Model file for the job. Use its own axes, mm. A direction names the side the tool comes from. Give positions to 0.01 mm unless a question says otherwise; leave off trailing zeros. Write each loop counter-clockwise with the first axis right and the second up, starting at its lowest first coordinate (ties: lowest second). Pieces come first, ordered by that corner, then holes. Notation, with made-up numbers: (59, 16) - (77, 16) arc R10 ccw to (77, 34) - close; hole circle Ø8 at (4.5, -14.5). An arc over 180 degrees is marked (long way). One line per item, written item: value. Start each with the question number.
(1) Drop flat-ended pins along their axis: P1, Ø4, axis at x = 0, z = 0.5, coming from the +Y side; P2, Ø1.2, axis at x = -1, z = 12.5, coming from the -Y side; P3, Ø2, axis at y = -2, z = 5.5, coming from the -X side. Give the stop position or say it passes through.
(2) Cut at C-C, the plane z = -4.25. List the corners of the cut face in (x, y), and give its area (3 significant figures).
(3) Cut at D-D, the plane y = 3.25. List the corners of the cut face in (x, z).
(4) Probe L1, parallel to Y at x = 1, z = 13.5; L2, parallel to Z at x = 3, y = 0.25; L3, parallel to Y at x = 0, z = 6.25. List the from-to ranges inside material, lowest first.
(5) Cut at B-B, the plane y = 0.75. List the corners of the cut face in (x, z).
(6) 3-axis set-ups, long thin cutter, end or side, ignore diameter. For faces 1 (the face through (0, 1.803, 15)), 2 (the face through (1, 3, 9.73)), 3 (the face through (0, -2, 10.73)): which of +Z, -Z, +X, -X, +Y, -Y reach the whole face in a straight line?
(7) Cut at A-A, the plane x = 0. List the corners of the cut face in (y, z), and give its area (3 significant figures).
from build123d import *

# Parameters (mm, degrees)
SKETCH1_R           = 2.7
BOSS_EXTRUDE1_DEPTH = 9.23
SKETCH2_R           = 3.6
BOSS_EXTRUDE2_DEPTH = 0.5
BOSS_EXTRUDE3_START = 1
SKETCH3_R           = 2.7
BOSS_EXTRUDE3_DEPTH = 1
BOSS_EXTRUDE4_START = 8.9
BOSS_EXTRUDE4_DEPTH = 8.9


with BuildPart() as part:
    # Sketch1 → Boss-Extrude1 (new, symmetric)
    with BuildSketch(Plane.XY):
        Circle(SKETCH1_R)
    extrude(amount=BOSS_EXTRUDE1_DEPTH, both=True)

    # Sketch2 → Boss-Extrude2 (add)
    with BuildSketch(Plane.XY.offset(9.23)):
        Circle(SKETCH2_R)
    extrude(amount=BOSS_EXTRUDE2_DEPTH)

    # Sketch3 → Boss-Extrude3 (add)
    with BuildSketch(Plane.XY.offset(9.73).offset(BOSS_EXTRUDE3_START)):
        Circle(SKETCH3_R)
    extrude(amount=-BOSS_EXTRUDE3_DEPTH)

    # Sketch3_3 → Boss-Extrude4 (add)
    with BuildSketch(Plane.XY.offset(9.73).offset(BOSS_EXTRUDE4_START)):
        with BuildLine():
            ThreePointArc((-2.01, 1.802747903), (-2.521606631, 0.965142477), (-2.7, 0))
            Line((-2.7, 0), (2.7, 0))
            ThreePointArc((2.7, 0), (2.521606631, 0.965142477), (2.01, 1.802747903))
            Line((2.01, 1.802747903), (-2.01, 1.802747903))
        make_face()
        with BuildLine():
            Line((2.7, 0), (-2.7, 0))
            ThreePointArc((-2.7, 0), (-2.521606631, -0.965142477), (-2.01, -1.802747903))
            Line((-2.01, -1.802747903), (2.01, -1.802747903))
            ThreePointArc((2.01, -1.802747903), (2.521606631, -0.965142477), (2.7, 0))
        make_face()
    extrude(amount=-BOSS_EXTRUDE4_DEPTH)


solid = part.part
Answers follow:
1. P1: stops at y = 2.7
1. P2: stops at y = -1.8
1. P3: stops at x = -2.51
2. outline: circle Ø5.4 at (0, 0)
2. area: 22.9 mm²
3. outline: (-1.55, 9.23) - (1.55, 9.23) - (1.55, 9.73) - (-1.55, 9.73) - close
4. L1: y = -1.8 to 1.8
4. L2: z = 9.23 to 9.73
4. L3: y = -2.7 to 2.7
5. outline: (-3.52, 9.23) - (-2.59, 9.23) - (-2.59, -9.23) - (2.59, -9.23) - (2.59, 9.23) - (3.52, 9.23) - (3.52, 9.73) - (2.59, 9.73) - (2.59, 18.63) - (-2.59, 18.63) - (-2.59, 9.73) - (-3.52, 9.73) - close
6. face 1: +Z, +X, -X, +Y
6. face 2: +Z
6. face 3: +Z, +X, -X, -Y
7. outline: (-3.6, 9.23) - (-2.7, 9.23) - (-2.7, -9.23) - (2.7, -9.23) - (2.7, 9.23) - (3.6, 9.23) - (3.6, 9.73) - (2.7, 9.73) - (2.7, 10.73) - (1.8, 10.73) - (1.8, 18.63) - (-1.8, 18.63) - (-1.8, 10.73) - (-2.7, 10.73) - (-2.7, 9.73) - (-3.6, 9.73) - close
7. area: 137 mm²
